Can you work these out from the drawing? Everything is in mm from the part's minimum corner. Round coordinates to 2 decimals unless told otherwise and drop trailing zeros. Write each loop counter-clockwise with the first axis right and the second up, starting at its lowest first coordinate (ties: lowest second). Pieces come first, ordered by that corner, then holes. Notation, with made-up numbers: M -31,-3 L 23,-3 A17 ccw 23,9 Z; hole C 62.25,-33.5 d2. An arc over 180 degrees is marked long. Use one line per item in the form item = value. Start each with the question number.
Q1. I need wall thicknesses on line 1 along X through (y, z) = (16.75, 0.7); line 2 along Y through (x, z) = (76.5, 1.3); line 3 along Y through (x, z) = (5, 2.25). Which ranges of each line are inside material? Lowest first, please. Write a range as from..to.
Q2. I want a section at B-B on z = 1.15. State how many separate pieces and enclosed holes the cut face has, and give its area (3 significant figures).
Q3. I'm going to push flat-ended pins straight in: pin 1 Ø0.8 at (y, z) = (15.5, 1) entering from -X; pin 2 Ø2 at (x, y) = (13.5, 15) entering from +Z. Where does each tip first touch, or does it pass through?
Q4. I want a section at A-A on x = 34.5. List the corners of the cut face in (y, z) for me, and give its area (3 significant figures).
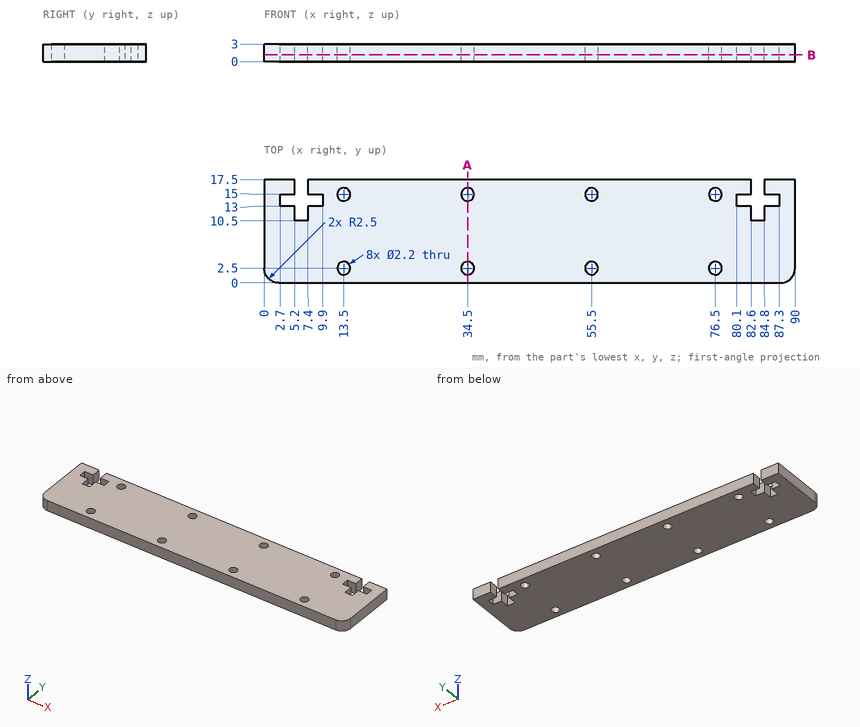
Reported:
q1.line_1 = 0..5.2, 7.4..82.6, 84.8..90
q1.line_2 = 0..1.4, 3.6..13.9, 16.1..17.5
q1.line_3 = 0..13, 15..17.5
q2.separate_pieces = 1
q2.enclosed_holes = 8
q2.area = 1,490 mm^2
q3.pin_1 = 0
q3.pin_2 = through
q4.outline = M 0,0 L 1.4,0 L 1.4,3 L 0,3 Z; M 3.6,0 L 13.9,0 L 13.9,3 L 3.6,3 Z; M 16.1,0 L 17.5,0 L 17.5,3 L 16.1,3 Z
q4.area = 39.3 mm^2
